Can you work these out from the model? Positions are in its coordinate system, mm. A direction names the side the tool comes from. Give positions to 0.01 mm unless a question says otherwise; leave off trailing zeros. Loops run counter-clockwise (first coordinate to the right, second up) from the corner with the lowest first, then second, coordinate; pieces in that order, holes last. Notation, with made-up numbers: (-7.75, -20) -> (43.25, -20) arc R16 ccw to (43.25, -9) -> close; hole circle Ø4 at (31.5, 62.25). An arc over 180 degrees is marked (long way). Return JSON: item names as keys, results as strings. Group by question number.
Q1. Suppose I cut it at A-A, the plane y = -3. Please give me the cut outline in (x, z), and give its area (3 significant figures).
Q2. Thinking about a two-plate mould opening in X: for faces 5 (the flat face through (0, 1.375, 4)), 6 (the flat face through (-4, -4, 0)), 7 (the flat face through (2.15, 0, 4)), which applies, pulls with the +X half, pulls with the -X half, needs draft (parallel to the pull), parting line crosses it, or undercut?
Q3. Suppose I cut it at C-C, the plane z = 1.5. Please give me the cut outline in (x, y) (3 decimals), and give its area (3 significant figures).
Q4. Will these pins go through, and if not, where does the flat tip stop? pin 1 (1.5 mm diameter, centred on x = 1.5, y = -2.5, fed in from +Z); pin 2 (2 mm diameter, centred on x = -1, z = 4, fed in from -Y) (3 decimals); pin 3 (2 mm diameter, centred on x = -1, z = -0.5, fed in from -Y).
Q5. Which directions (+Z, -Z, +X, -X, +Y, -Y) give clear straight access to the entire face, cutting with the end or side of a thin tool? Please do faces 1 (the flat face through (0, -0.625, 4)), 2 (the flat face through (0, -2.375, -1)), 3 (the flat face through (-2.15, 0, 4)), 4 (the flat face through (4, -4, 0)).
Q6. I need wall thicknesses on line 1 along X through (y, z) = (-2.75, 0.25); line 2 along Z through (x, y) = (2, -1); line 3 along Y through (x, z) = (0.75, 4.5) (3 decimals). Which ranges of each line are inside material? Lowest first, please. Write a range as [from, to].
Autodesk Inventor part; units mm, degrees
ref_plane "Work Plane1" through (0, -0.625, 2.25) normal (1, 0, 0) x (0, 0, -1)
ref_plane "YZ Plane" through (0, 0, 0) normal (1, 0, 0) x (0, 1, 0)
ref_plane "XY Plane" through (0, 0, 0) normal (0, 0, 1) x (1, 0, 0)
sketch "Sketch1" plane through (0, 0, 0) normal (0, 0, 1) x (1, 0, 0)
  line L0 (-4.4, 2.375) -> (4.4, 2.375)
  line L1 (4.4, 2.375) -> (4.4, -2.375)
  line L2 (4.4, -2.375) -> (-4.4, -2.375)
  line L3 (-4.4, -2.375) -> (-4.4, 2.375)
  line L4 (-6.16, 0) -> (6.16, 0) construction
  line L5 (0, -3.325) -> (0, 3.325) construction
  point P0 (0, 0)
  dimension "d0" = 8.8
  dimension "d1" = 4.75
extrude "Extrusion1" add sketch "Sketch1" along normal mid plane 4.5
sketch "Sketch2" plane through (0, 0, 2.25) normal (0, 0, 1) x (1, 0, 0)
  line L0 (-2.15, 1.375) -> (2.15, 1.375)
  line L1 (2.15, 1.375) -> (2.15, -0.625)
  line L2 (2.15, -0.625) -> (-2.15, -0.625)
  line L3 (-2.15, -0.625) -> (-2.15, 1.375)
  line L4 (0, -3.325) -> (0, 3.325) construction
  line L5 (-6.16, 0) -> (6.16, 0) construction
  line L6 (4.4, 2.375) -> (-4.4, 2.375)
  point P0 (0, 0)
  dimension "d4" = 4.3
  dimension "d5" = 2
  dimension "d30" = 1
extrude "Extrusion2" add sketch "Sketch2" along normal blind 3
ref_plane "Work Plane1" through (0, -0.625, 2.25) normal (1, 0, 0) x (0, 0, -1)
split_face "Split1"
sketch "Sketch6" plane through (-2.15, 1.375, 2.25) normal (0, 1, 0) x (1, 0, 0)
  line L0 (2.15, -3) -> (0, -3)
  line L1 (0.5375, -3) -> (1.075, -2.4625)
  line L2 (1.075, -2.4625) -> (1.6125, -3)
  line L3 (0, -3) -> (2.15, -3)
  point P0 (2.15, 2.25)
  point P1 (1.075, -3)
  point P2 (1.075, -3)
  dimension "d24" = 2.15
  dimension "d25" = 0.5375
  dimension "d26" = 45
extrude "Extrusion4" cut sketch "Sketch6" against normal up to surface (2 mm away)
mirror "Mirror1" about plane through (0, -0.625, 2.25) normal (1, 0, 0) of "Extrusion4"
sketch "Sketch3" plane through (-4.4, -2.375, 2.25) normal (0, -1, 0) x (1, 0, 0)
  line L0 (0, -4.5) -> (0, 0) construction
  line L1 (0, -1.65) -> (0.4, -1.65)
  line L2 (0.4, -1.65) -> (0.4, -2.85)
  line L3 (0.4, -2.85) -> (0, -2.85)
  line L4 (0, -2.85) -> (0, -1.65)
  line L5 (8.8, -4.5) -> (8.8, 0) construction
  line L6 (8.8, -1.65) -> (8.4, -1.65)
  line L7 (8.4, -1.65) -> (8.4, -2.85)
  line L8 (8.4, -2.85) -> (8.8, -2.85)
  line L9 (8.8, -2.85) -> (8.8, -1.65)
  line L10 (4.15, -2.1) -> (4.65, -2.1)
  line L11 (4.65, -2.1) -> (4.65, -2.4)
  line L12 (4.65, -2.4) -> (4.15, -2.4)
  line L13 (4.15, -2.4) -> (4.15, -2.1)
  line L14 (2.15, -2.1) -> (2.65, -2.1)
  line L15 (2.65, -2.1) -> (2.65, -2.4)
  line L16 (2.65, -2.4) -> (2.15, -2.4)
  line L17 (2.15, -2.4) -> (2.15, -2.1)
  line L18 (6.15, -2.1) -> (6.65, -2.1)
  line L19 (6.65, -2.1) -> (6.65, -2.4)
  line L20 (6.65, -2.4) -> (6.15, -2.4)
  line L21 (6.15, -2.4) -> (6.15, -2.1)
  line L22 (-1.76, -2.25) -> (10.56, -2.25) construction
  line L23 (4.4, -6) -> (4.4, 4.5) construction
  point P0 (4.4, -2.25)
  dimension "d8" = 0.4
  dimension "d9" = 1.2
  dimension "d10" = 0.4
  dimension "d11" = 0.5
  dimension "d12" = 0.3
  dimension "d13" = 0.5
  dimension "d14" = 0.3
  dimension "d15" = 0.5
  dimension "d16" = 0.3
  dimension "d17" = 1.5
extrude "Extrusion3" add sketch "Sketch3" along normal blind 2.6
fillet "Fillet1" radius 0.6 4 edges at (4.2, -4.975, 0.6) (4.2, -4.975, -0.6) (-4.2, -4.975, -0.6) (-4.2, -4.975, 0.6)
fillet "Fillet2" radius 0.25 6 edges at (2.25, -4.975, 0) (1.75, -4.975, 0) (0.25, -4.975, 0) (-0.25, -4.975, 0) (-1.75, -4.975, 0) (-2.25, -4.975, 0)
fillet "Fillet3" radius 0.5 4 edges at (4.4, 2.375, 0) (-4.4, 2.375, 0) (0, 2.375, 2.25) (0, 2.375, -2.25)
properties part number "Power_switch"
Ans:
{
 "1": {"outline": "(-4.4, -0.6) -> (-4, -0.6) -> (-4, 0.6) -> (-4.4, 0.6) -> close; (-2.25, -0.15) -> (-1.75, -0.15) -> (-1.75, 0.15) -> (-2.25, 0.15) -> close; (-0.25, -0.15) -> (0.25, -0.15) -> (0.25, 0.15) -> (-0.25, 0.15) -> close; (1.75, -0.15) -> (2.25, -0.15) -> (2.25, 0.15) -> (1.75, 0.15) -> close; (4, -0.6) -> (4.4, -0.6) -> (4.4, 0.6) -> (4, 0.6) -> close", "area": "1.41 mm^2"},
 "2": {"face 5": "needs draft", "face 6": "undercut", "face 7": "pulls with the +X half"},
 "3": {"outline": "(-4.4, -2.375) -> (4.4, -2.375) -> (4.4, 1.875) arc R0.5 ccw to (3.9, 2.375) -> (-3.9, 2.375) arc R0.5 ccw to (-4.4, 1.875) -> close", "area": "41.7 mm^2"},
 "4": {"pin 1": "stops at z = 2.25", "pin 2": "stops at y = -0.625", "pin 3": "stops at y = -4.97"},
 "5": {"face 1": "+Z, +X, -X, -Y", "face 2": "-Y", "face 3": "+Z, -X, +Y, -Y", "face 4": "+Z, -Z, -Y"},
 "6": {"line 1": "x = [-4.4, -4], [4, 4.4]", "line 2": "z = [-2.25, 2.25]", "line 3": "y = [-0.625, 1.375]"}
}
